from build123d import *

# Parameters (mm, degrees)
BOSS_EXTRUDE1_DEPTH = 2
FILLET1_R           = 0.5


with BuildPart() as part:
    # Sketch1 → Boss-Extrude1 (new body)
    with BuildSketch(Plane(origin=(0, 0, 0), x_dir=(1, 0, 0), z_dir=(0, 1, 0))):
        with BuildLine():
            Line((-0.5, 4), (-4, 4))
            Line((-4, 4), (-4, 0.5))
            Line((-4, 0.5), (-2.866025404, 0.5))
            ThreePointArc((-2.866025404, 0.5), (-1.741180955, 0.965925826), (-1, 0))
            ThreePointArc((-1, 0), (-1.741180955, -0.965925826), (-2.866025404, -0.5))
            Line((-2.866025404, -0.5), (-4, -0.5))
            Line((-4, -0.5), (-4, -4))
            Line((-4, -4), (-0.5, -4))
            Line((-0.5, -4), (-0.5, -2.866025404))
            ThreePointArc((-0.5, -2.866025404), (-0.5, -1.133974596), (1, -2))
            ThreePointArc((1, -2), (0.866025404, -2.5), (0.5, -2.866025404))
            Line((0.5, -2.866025404), (0.5, -4))
            Line((0.5, -4), (4, -4))
            Line((4, -4), (4, -0.5))
            Line((4, -0.5), (2.866025404, -0.5))
            ThreePointArc((2.866025404, -0.5), (1, 0), (2.866025404, 0.5))
            Line((2.866025404, 0.5), (4, 0.5))
            Line((4, 0.5), (4, 4))
            Line((4, 4), (0.5, 4))
            Line((0.5, 4), (0.5, 2.866025404))
            ThreePointArc((0.5, 2.866025404), (0.866025404, 2.5), (1, 2))
            ThreePointArc((1, 2), (-0.5, 1.133974596), (-0.5, 2.866025404))
            Line((-0.5, 2.866025404), (-0.5, 4))
        make_face()
    extrude(amount=BOSS_EXTRUDE1_DEPTH)

    # Fillet1
    fillet1_edges = [part.edges().sort_by_distance(p)[0] for p in [
        (-2.866025404, 1, -0.5),
        (-4, 1, -0.5),
        (-0.5, 1, -4),
        (-0.5, 1, -2.866025404),
        (0.5, 1, -2.866025404),
        (0.5, 1, -4),
        (4, 1, -0.5),
        (2.866025404, 1, -0.5),
        (2.866025404, 1, 0.5),
        (4, 1, 0.5),
        (0.5, 1, 4),
        (0.5, 1, 2.866025404),
        (-0.5, 1, 2.866025404),
        (-0.5, 1, 4),
        (-4, 1, 0.5),
        (-2.866025404, 1, 0.5),
    ]]
    fillet(fillet1_edges, radius=FILLET1_R)


solid = part.part
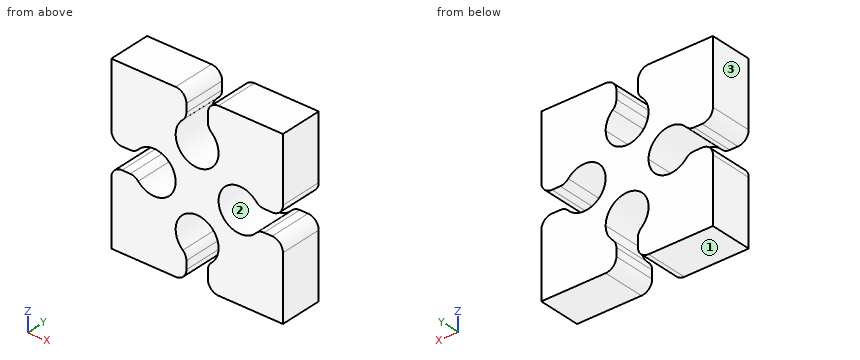
Work out the finished part from the listing and answer in its coordinate system (mm). Face numbers are marked on the shaded views. Round coordinates to 2 decimals unless told otherwise and drop trailing zeros. Loops run counter-clockwise (first coordinate to the right, second up) from the corner with the lowest first, then second, coordinate; pieces in that order, holes last. Notation, with made-up numbers: (21, 27.25) - (57, 27.25) arc R34 ccw to (57, 65.25) - close; hole circle Ø1 at (89, -3.5). An arc over 180 degrees is marked (long way). Use one line per item in the form item = value. Start each with the question number.
(1) Find section C-C on x = 0. Determine the outline of the cut face in (y, z), and give its area (3 significant figures).
(2) A flat-ended cylindrical pin translates along its axis: P1, Ø1.6, axis at x = 2, z = 0, coming from the -Y side. Find the tip coordinate at first contact, or state that the pin passes through.
(3) Find section B-B on z = 3.25. Determine the outline of the cut face in (x, y).
(4) Consider line 1 (X direction, y = 1.1, z = -2); line 2 (X direction, y = 1.4, z = -0.75); line 3 (Z direction, x = -3.25, y = 1.2). Determine where each line is inside the solid, lowest interval first.
(5) Find section A-A on x = 2. Determine the outline of the cut face in (y, z).
(6) Determine the mould class of the marked faces 1, 2 and 3 for opening direction Z: +Z half, -Z half, draft (parallel to the pull), parting line (faces both ways), or undercut.
Answer list:
q1.outline = (0, -1) - (2, -1) - (2, 1) - (0, 1) - close
q1.area = 4.00 mm^2
q2.P1 = through
q3.outline = (-4, 0) - (-0.5, 0) - (-0.5, 2) - (-4, 2) - close; (0.5, 0) - (4, 0) - (4, 2) - (0.5, 2) - close
q4.line_1 = -4 to -1, 1 to 4
q4.line_2 = -3.93 to -2.66, -1.34 to 1.34, 2.66 to 3.93
q4.line_3 = -4 to -0.5, 0.5 to 4
q5.outline = (0, -4) - (2, -4) - (2, -1) - (0, -1) - close; (0, 1) - (2, 1) - (2, 4) - (0, 4) - close
q6.face_1 = -Z half
q6.face_2 = undercut
q6.face_3 = draft
